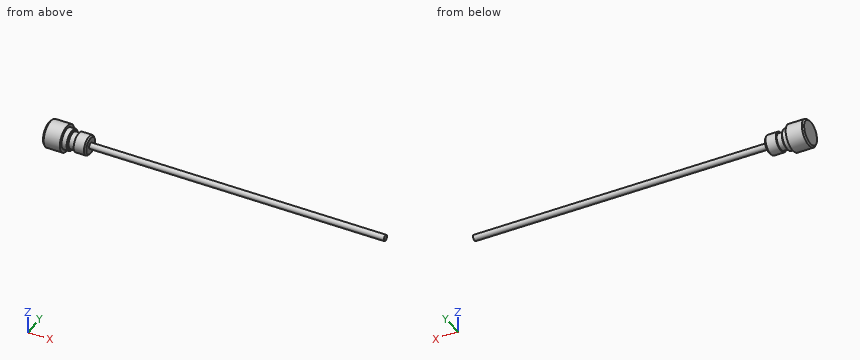
```python
from build123d import *

# Parameters (mm, degrees)
CROQUIS1_R              = 9
SALIENTE_EXTRUIR1_DEPTH = 12
CHAFL_N1_SIZE           = 1
CROQUIS2_R              = 7
SALIENTE_EXTRUIR2_DEPTH = 4
CROQUIS3_R              = 5.5
SALIENTE_EXTRUIR3_DEPTH = 4
CROQUIS4_R              = 6.5
SALIENTE_EXTRUIR4_DEPTH = 8
CHAFL_N2_SIZE           = 1
CROQUIS5_R              = 2
SALIENTE_EXTRUIR5_DEPTH = 200
CHAFL_N3_SIZE           = 0.5


with BuildPart() as part:
    # Croquis1 → Saliente-Extruir1 (new body)
    with BuildSketch(Plane(origin=(0, 0, 0), x_dir=(0, 0, -1), z_dir=(1, 0, 0))):
        Circle(CROQUIS1_R)
    extrude(amount=SALIENTE_EXTRUIR1_DEPTH)

    # Chaflán1
    chafl_n1_edges = [part.edges().sort_by_distance(p)[0] for p in [
        (0, 0, 9),
    ]]
    chamfer(chafl_n1_edges, length=CHAFL_N1_SIZE)

    # Croquis2 → Saliente-Extruir2 (add)
    with BuildSketch(Plane(origin=(12, 0, 0), x_dir=(0, 0, -1), z_dir=(1, 0, 0))):
        Circle(CROQUIS2_R)
    extrude(amount=SALIENTE_EXTRUIR2_DEPTH)

    # Croquis3 → Saliente-Extruir3 (add)
    with BuildSketch(Plane(origin=(16, 0, 0), x_dir=(0, 0, -1), z_dir=(1, 0, 0))):
        Circle(CROQUIS3_R)
    extrude(amount=SALIENTE_EXTRUIR3_DEPTH)

    # Croquis4 → Saliente-Extruir4 (add)
    with BuildSketch(Plane(origin=(20, 0, 0), x_dir=(0, 0, -1), z_dir=(1, 0, 0))):
        Circle(CROQUIS4_R)
    extrude(amount=SALIENTE_EXTRUIR4_DEPTH)

    # Chaflán2
    chafl_n2_edges = [part.edges().sort_by_distance(p)[0] for p in [
        (28, 0, 6.5),
    ]]
    chamfer(chafl_n2_edges, length=CHAFL_N2_SIZE)

    # Croquis5 → Saliente-Extruir5 (add)
    with BuildSketch(Plane(origin=(28, 0, 0), x_dir=(0, 0, -1), z_dir=(1, 0, 0))):
        Circle(CROQUIS5_R)
    extrude(amount=SALIENTE_EXTRUIR5_DEPTH)

    # Chaflán3
    chafl_n3_edges = [part.edges().sort_by_distance(p)[0] for p in [
        (16, 0, 7),
    ]]
    chamfer(chafl_n3_edges, length=CHAFL_N3_SIZE)


solid = part.part
```
Design review of the part built by this model. Coordinates are the model's own, in mm. Round coordinates to 2 decimals unless told otherwise and drop trailing zeros. Write each loop counter-clockwise with the first axis right and the second up, starting at its lowest first coordinate (ties: lowest second). Pieces come first, ordered by that corner, then holes. Notation, with made-up numbers: (81, 56.5) -> (93, 56.5) arc R16 cw to (93, 69.5) -> close; hole circle Ø2 at (65, -10). An arc over 180 degrees is marked (long way). Write item = value, one per line. Start each with the question number.
1) Clearance check with flat-ended pins moving along their axes: pin 1 (1 mm diameter, centred on y = -3, z = -3.5, fed in from +X); pin 2 (6 mm diameter, centred on x = 158, y = 0, fed in from -Z); pin 3 (4 mm diameter, centred on x = 164.5, z = -2, fed in from -Y). State where each tip first meets the part, or that it passes through.
2) Wall thickness on probe 1 along Z at (x, y) = (25, 0.25); probe 2 along X at (y, z) = (-4, 6.5); probe 3 along X at (y, z) = (3.75, 0): over which ranges is each line inside the solid? List them lowest first. Write a range as from..to.
3) Take a section at C-C, the plane x = 84. State the section outline as (y, z) points, plus the area to 3 significant figures.
4) Take a section at A-A, the plane y = 0. State the section outline as (x, z) points.
Results list:
q1.pin_1 = 28
q1.pin_2 = -2
q1.pin_3 = -2
q2.probe_1 = -6.5..6.5
q2.probe_2 = 0..12
q2.probe_3 = 0..28
q3.outline = circle Ø4 at (0, 0)
q3.area = 12.6 mm²
q4.outline = (0, -8) -> (1, -9) -> (12, -9) -> (12, -7) -> (15.5, -7) -> (16, -6.5) -> (16, -5.5) -> (20, -5.5) -> (20, -6.5) -> (27, -6.5) -> (28, -5.5) -> (28, -2) -> (228, -2) -> (228, 2) -> (28, 2) -> (28, 5.5) -> (27, 6.5) -> (20, 6.5) -> (20, 5.5) -> (16, 5.5) -> (16, 6.5) -> (15.5, 7) -> (12, 7) -> (12, 9) -> (1, 9) -> (0, 8) -> close
